For this review, take the finished solid that the model builds, in its own axes (mm). A direction names the side the tool comes from. Coordinates: 2 decimals unless noted, no trailing zeros. Write each loop counter-clockwise with the first axis right and the second up, starting at its lowest first coordinate (ties: lowest second). Pieces come first, ordered by that corner, then holes. Notation, with made-up numbers: M 35,76.25 L 56,76.25 A13 ccw 56,101.25 Z; hole C -39,48.5 d5. An arc over 180 degrees is marked long. One line per question, with ' | ' between items.
from build123d import *

# Parameters (mm, degrees)
SKETCH1_W           = 180
SKETCH1_H           = 78
BOSS_EXTRUDE1_DEPTH = 75
SKETCH7_W           = 170
SKETCH7_H           = 68
CUT_EXTRUDE1_DEPTH  = 70
SKETCH8_W           = 68
SKETCH8_H           = 65
CUT_EXTRUDE2_DEPTH  = 5
SKETCH2_R           = 5.5
SKETCH2_R_2         = 6
CUT_EXTRUDE3_DEPTH  = 5
SKETCH6_R           = 5.5
CUT_EXTRUDE5_DEPTH  = 5
SKETCH9_W           = 10
SKETCH9_H           = 10
BOSS_EXTRUDE2_DEPTH = 6


with BuildPart() as part:
    # Sketch1 → Boss-Extrude1 (new body)
    with BuildSketch(Plane(origin=(0, 0, 0), x_dir=(1, 0, 0), z_dir=(0, 1, 0))):
        with Locations((90, -39)):
            Rectangle(SKETCH1_W, SKETCH1_H)
    extrude(amount=BOSS_EXTRUDE1_DEPTH)

    # Sketch7 → Cut-Extrude1 (cut)
    with BuildSketch(Plane(origin=(0, 0, 0), x_dir=(1, 0, 0), z_dir=(0, 1, 0))):
        with Locations((90, -39)):
            Rectangle(SKETCH7_W, SKETCH7_H)
    extrude(amount=CUT_EXTRUDE1_DEPTH, mode=Mode.SUBTRACT)

    # Sketch8 → Cut-Extrude2 (cut)
    with BuildSketch(Plane(origin=(180, 0, 0), x_dir=(0, 0, -1), z_dir=(1, 0, 0))):
        with Locations((-39, 37.5)):
            Rectangle(SKETCH8_W, SKETCH8_H)
    extrude(amount=-CUT_EXTRUDE2_DEPTH, mode=Mode.SUBTRACT)

    # Sketch2 → Cut-Extrude3 (cut)
    with BuildSketch(Plane.XY.offset(78)):
        with Locations((160.21219032, 25)):
            Circle(SKETCH2_R)
        with Locations((100.21219032, 25)):
            Circle(SKETCH2_R)
        with Locations((130.21219032, 25)):
            Circle(SKETCH2_R)
        with Locations((70.21219032, 25)):
            Circle(SKETCH2_R)
        with Locations((33.219063995, 44.738868471)):
            Circle(SKETCH2_R_2)
        with Locations((33.219063995, 15.81956505)):
            Circle(SKETCH2_R_2)
    extrude(amount=-CUT_EXTRUDE3_DEPTH, mode=Mode.SUBTRACT)

    # Sketch6 → Cut-Extrude5 (cut)
    with BuildSketch(Plane(origin=(0, 0, 0), x_dir=(0, 0, -1), z_dir=(1, 0, 0))):
        with Locations((-46.363872843, 44.63646506)):
            Circle(SKETCH6_R)
        with Locations((-46.363872843, 15.486690828)):
            Circle(SKETCH6_R)
    extrude(amount=CUT_EXTRUDE5_DEPTH, mode=Mode.SUBTRACT)

    # Sketch9 → Boss-Extrude2 (add)
    with BuildSketch(Plane(origin=(0, 0, 73), x_dir=(-1, 0, 0), z_dir=(0, 0, -1))):
        with Locations((-175, 60)):
            Rectangle(SKETCH9_W, SKETCH9_H)
        with Locations((-90, 60)):
            Rectangle(SKETCH9_W, SKETCH9_H)
        with Locations((-10, 60)):
            Rectangle(SKETCH9_W, SKETCH9_H)
    boss_extrude2 = extrude(amount=BOSS_EXTRUDE2_DEPTH)

    # Mirror1: Boss-Extrude2 across plane
    add(boss_extrude2.mirror(Plane.XY.offset(39)))


solid = part.part
1. Draft analysis for pull direction Y (two halves, no side actions). For faces 4 (the cylindrical face through (38.76, 13.52, 75.54)), 5 (the flat face through (90, 55, 8)), 6 (the flat face through (170, 60, 8)), 7 (the flat face through (175, 65, 8)), state which applies: pulls with the +Y half, pulls with the -Y half, needs draft (parallel to the pull), parting line crosses it, or undercut.
Computed values:
face 4: undercut | face 5: pulls with the -Y half | face 6: needs draft | face 7: undercut
2. Clearance check with flat-ended pins moving along their axes: P1, Ø2, axis at y = 24.5, z = 56.5, coming from the +X side; P2, Ø5, axis at x = 47.5, z = 63.5, coming from the -Y side; P3, Ø9, axis at y = 15.49, z = 46.36, coming from the -X side (3 decimals); P4, Ø1.8, axis at x = 89, z = 8, coming from the -Y side. State where each tip first meets the part, or that it passes through.
Computed values:
P1: stops at x = 5 | P2: stops at y = 70 | P3: passes through | P4: stops at y = 55
3. Take a section at D-D on z = 46.5. State the section outline as (x, y) points (3 decimals), plus the area to 3 significant figures.
Computed values:
outline: M 0,0 L 5,0 L 5,9.988 L 0,9.988 Z; M 0,20.985 L 5,20.985 L 5,39.138 L 0,39.138 Z; M 0,50.135 L 5,50.135 L 5,70 L 180,70 L 180,75 L 0,75 Z; M 175,0 L 180,0 L 180,5 L 175,5 Z | area: 1,170 mm2
4. For line 1 along Z through (x, y) = (160, 37); line 2 along Y through (x, z) = (16, 66); line 3 along Z through (x, y) = (34, 10.5), list the stretches that pass through material, from the lowest coordinate up.
Computed values:
line 1: z = 0 to 5, 73 to 78 | line 2: y = 70 to 75 | line 3: z = 0 to 5
5. Take a section at A-A on z = 25.5. State the section outline as (x, y) points, plus the area to 4 significant figures.
Computed values:
outline: M 0,0 L 5,0 L 5,70 L 180,70 L 180,75 L 0,75 Z; M 175,0 L 180,0 L 180,5 L 175,5 Z | area: 1,275 mm2
6. Take a section at C-C on x = 149. State the section outline as (y, z) points.
Computed values:
outline: M 0,0 L 75,0 L 75,78 L 0,78 L 0,73 L 70,73 L 70,5 L 0,5 Z
7. Take a section at B-B on y = 25. State the section outline as (x, z) points.
Computed values:
outline: M 0,0 L 180,0 L 180,5 L 5,5 L 5,73 L 64.71,73 L 64.71,78 L 0,78 Z; M 75.71,73 L 94.71,73 L 94.71,78 L 75.71,78 Z; M 105.71,73 L 124.71,73 L 124.71,78 L 105.71,78 Z; M 135.71,73 L 154.71,73 L 154.71,78 L 135.71,78 Z; M 165.71,73 L 180,73 L 180,78 L 165.71,78 Z
8. Machinability: for faces 1 (the flat face through (175, 55, 8)), 2 (the flat face through (10, 60, 11)), 3 (the cylindrical face through (75.46, 26.65, 75.54)), which of the approach directions +Z, -Z, +X, -X, +Y, -Y give a long, thin tool a straight path to every point of the face, cutting with its end or side? Answer none if there is none.
Computed values:
face 1: +X | face 2: +X, -Y | face 3: +Z
